Input: part model. Units: mm. Frame: model coordinates. A direction names the side the tool comes from. Coordinates: 2 decimals unless noted, no trailing zeros. Order: outer loops, then holes, each group sorted by start corner. A loop starts at its lowest first (then second) coordinate and runs counter-clockwise, first axis right, second up. Notation, with made-up numbers: (30.5, 6.25) -> (40.5, 6.25) arc R18 cw to (40.5, 16.25) -> close; hole circle Ø8 at (74, -30). An arc over 180 degrees is marked (long way). One line per question, with ' | ' between items.
```python
from build123d import *

# Parameters (mm, degrees)
F1_DEPTH      = 113
F2_R          = 6.5
F3_DEPTH      = 113.001
F4_W          = 35
F4_H          = 17
F5_DEPTH      = 32.001
F6_W          = 25
F6_H          = 51
F7_DEPTH      = 16.001
F7_DEPTH_BACK = 16.001
F8_R          = 5.5
F9_DEPTH      = 29.001


with BuildPart() as f1:
    # F0 (on Right) → F1 (new body)
    with BuildSketch(Plane.YZ):
        with BuildLine():
            ThreePointArc((16, 31.128765), (0, 35), (-16, 31.128765))
            Line((-16, 31.128765), (-16, -29))
            Line((-16, -29), (16, -29))
            Line((16, -29), (16, 31.128765))
        make_face()
    extrude(amount=F1_DEPTH)

    # F2 (on face) → F3 (cut, through all)
    with BuildSketch(Plane.YZ.offset(113)):
        with Locations((0, 17)):
            Circle(F2_R)
    extrude(amount=-F3_DEPTH, mode=Mode.SUBTRACT)

    # F4 (on face) → F5 (cut, through all)
    with BuildSketch(Plane.XZ.offset(16)):
        with Locations((56.5, -20.5)):
            Rectangle(F4_W, F4_H)
        Polygon((44, 1), (69, 1), (69.100894, 35.176743), (44, 35.176743), align=None)
    extrude(amount=-F5_DEPTH, mode=Mode.SUBTRACT)

    # F6 (on Front) → F7 (cut, two sides)
    with BuildSketch(Plane.XZ) as f7_sk:
        with Locations((12.5, 9.5)):
            Rectangle(F6_W, F6_H)
        with Locations((100.550447, 9.5)):
            Rectangle(F6_W, F6_H)
    extrude(amount=F7_DEPTH, mode=Mode.SUBTRACT)
    extrude(f7_sk.sketch, amount=-F7_DEPTH_BACK, mode=Mode.SUBTRACT)

    # F8 (on Top) → F9 (cut, through all)
    with BuildSketch(Plane.XY):
        Polygon((10, -16), (0, -6), (0, -16), align=None)
        with Locations((13, 0)):
            Circle(F8_R)
        with Locations((100, 0)):
            Circle(F8_R)
        Polygon((113, -6), (103, -16), (113, -16), align=None)
    extrude(amount=-F9_DEPTH, mode=Mode.SUBTRACT)


solid = f1.part
```
1. Cut plane A-A, the plane z = -24.5. Return loops of the section in (x, y).
Recorded:
outline: (0, -6) -> (10, -16) -> (39, -16) -> (39, 16) -> (0, 16) -> close; (74, -16) -> (103, -16) -> (113, -6) -> (113, 16) -> (74, 16) -> close; hole circle Ø11 at (13, 0); hole circle Ø11 at (100, 0)
2. Ray query, line 1 (Y direction, x = 100, z = -23.75); line 2 (X direction, y = 8.5, z = -18); line 3 (Z direction, x = 35.25, y = 0). Return the intervals inside material, ascending. Write a range as [from, to].
Recorded:
line 1: y = [-16, -5.5], [5.5, 16] | line 2: x = [0, 39], [74, 113] | line 3: z = [-29, 10.5], [23.5, 35]
3. Mould query, pull axis Y, two halves, no side actions, for faces 6 (the face through (34, 0, 35)), 7 (the face through (74, 0, -21)), 8 (the face through (78.67, -0.846, 23.445)). Classes: released by +Y, released by -Y, zero draft, split by the parting line, or undercut.
Recorded:
face 6: split by the parting line | face 7: zero draft | face 8: undercut
4. Cut plane C-C, the plane z = 17. Return loops of the section in (x, y), and give its area (3 significant figures).
Recorded:
outline: (25, -16) -> (44, -16) -> (44, -6.5) -> (25, -6.5) -> close; (25, 6.5) -> (44, 6.5) -> (44, 16) -> (25, 16) -> close; (69.05, -16) -> (88.05, -16) -> (88.05, -6.5) -> (69.05, -6.5) -> close; (69.05, 6.5) -> (88.05, 6.5) -> (88.05, 16) -> (69.05, 16) -> close | area: 722 mm^2
5. Access query for faces 1 (the face through (56, 0, 1)), 2 (the face through (39, 0, -21)), 3 (the face through (95, 4, -16)), 4 (the face through (113, 5, -22)), 5 (the face through (93, 0, -29)). Directions: +Z, -Z, +X, -X, +Y, -Y. A direction counts if a zero-diameter tool reaches every point of the face in a straight line with its end or side. Return the directions, or none.
Recorded:
face 1: +Z, +Y, -Y | face 2: -Z, +Y, -Y | face 3: +Z, +X, +Y, -Y | face 4: +Z, -Z, +X, +Y, -Y | face 5: -Z, +X, -X, +Y, -Y
6. Cut plane D-D, the plane z = 3. Return loops of the section in (x, y).
Recorded:
outline: (25, -16) -> (44, -16) -> (44, 16) -> (25, 16) -> close; (69.01, -16) -> (88.05, -16) -> (88.05, 16) -> (69.01, 16) -> close
7. Pin query (flat end, axial travel): pin 1 Ø12 at (x, y) = (12.5, 9.5) entering from +Z; pin 2 Ø13.5 at (y, z) = (-0.5, -19.5) entering from -X; pin 3 Ø16 at (y, z) = (-4, 22.5) entering from +X; pin 4 Ø6 at (x, y) = (33, 7) entering from +Z. Return the tip coordinate at first contact, or that it passes through.
Recorded:
pin 1: stops at z = -16 | pin 2: stops at x = 0 | pin 3: stops at x = 88.05 | pin 4: stops at z = 34.77
8. Cut plane B-B, the plane x = 13. Return loops of the section in (y, z), and give its area (3 significant figures).
Recorded:
outline: (-16, -29) -> (-5.5, -29) -> (-5.5, -16) -> (-16, -16) -> close; (5.5, -29) -> (16, -29) -> (16, -16) -> (5.5, -16) -> close | area: 273 mm^2
